from build123d import *

# Parameters (mm, degrees)
SKETCH1_W           = 164
SKETCH1_H           = 55
SKETCH1_W_2         = 15
SKETCH1_H_2         = 2.5
BOSS_EXTRUDE1_DEPTH = 3
CUT_EXTRUDE1_DEPTH  = 3
SKETCH3_R           = 1.25
CUT_EXTRUDE2_DEPTH  = 10
SKETCH4_R           = 2.5
CUT_EXTRUDE3_DEPTH  = 4
SKETCH5_R           = 1.5
CUT_EXTRUDE4_DEPTH  = 10


with BuildPart() as part:
    # Sketch1 → Boss-Extrude1 (new body)
    with BuildSketch(Plane(origin=(0, 0, 0), x_dir=(1, 0, 0), z_dir=(0, 1, 0))):
        Rectangle(SKETCH1_W, SKETCH1_H)
        with Locations((48.5, 14.5)):
            Rectangle(SKETCH1_W_2, SKETCH1_H_2, mode=Mode.SUBTRACT)
        with Locations((68.5, 14.5)):
            Rectangle(SKETCH1_W_2, SKETCH1_H_2, mode=Mode.SUBTRACT)
        with Locations((68.5, -14.5)):
            Rectangle(SKETCH1_W_2, SKETCH1_H_2, mode=Mode.SUBTRACT)
        with Locations((48.5, -14.5)):
            Rectangle(SKETCH1_W_2, SKETCH1_H_2, mode=Mode.SUBTRACT)
        with Locations((-48.5, -14.5)):
            Rectangle(SKETCH1_W_2, SKETCH1_H_2, mode=Mode.SUBTRACT)
        with Locations((-68.5, -14.5)):
            Rectangle(SKETCH1_W_2, SKETCH1_H_2, mode=Mode.SUBTRACT)
        with Locations((-68.5, 14.5)):
            Rectangle(SKETCH1_W_2, SKETCH1_H_2, mode=Mode.SUBTRACT)
        with Locations((-48.5, 14.5)):
            Rectangle(SKETCH1_W_2, SKETCH1_H_2, mode=Mode.SUBTRACT)
    extrude(amount=BOSS_EXTRUDE1_DEPTH)

    # Sketch2 → Cut-Extrude1 (cut)
    with BuildSketch(Plane(origin=(0, 3, 0), x_dir=(1, 0, 0), z_dir=(0, 1, 0))):
        with BuildLine():
            Line((-31.658505885, 2), (-8.266387648, 2))
            ThreePointArc((-8.266387648, 2), (-6.266387648, 0), (-8.266387648, -2))
            Line((-8.266387648, -2), (-31.658505885, -2))
            ThreePointArc((-31.658505885, -2), (-33.658505885, 0), (-31.658505885, 2))
        make_face()
        with BuildLine():
            Line((31.658505885, -9.856733432), (8.266387648, -9.856733432))
            ThreePointArc((8.266387648, -9.856733432), (6.266387648, -7.856733432), (8.266387648, -5.856733432))
            Line((8.266387648, -5.856733432), (31.658505885, -5.856733432))
            ThreePointArc((31.658505885, -5.856733432), (33.658505885, -7.856733432), (31.658505885, -9.856733432))
        make_face()
        with BuildLine():
            Line((-31.658505885, 9.620758334), (-8.266387648, 9.620758334))
            ThreePointArc((-8.266387648, 9.620758334), (-6.266387648, 7.620758334), (-8.266387648, 5.620758334))
            Line((-8.266387648, 5.620758334), (-31.658505885, 5.620758334))
            ThreePointArc((-31.658505885, 5.620758334), (-33.658505885, 7.620758334), (-31.658505885, 9.620758334))
        make_face()
        with BuildLine():
            Line((31.658505885, 5.620758334), (8.266387648, 5.620758334))
            ThreePointArc((8.266387648, 5.620758334), (6.266387648, 7.620758334), (8.266387648, 9.620758334))
            Line((8.266387648, 9.620758334), (31.658505885, 9.620758334))
            ThreePointArc((31.658505885, 9.620758334), (33.658505885, 7.620758334), (31.658505885, 5.620758334))
        make_face()
        with BuildLine():
            Line((-31.658505885, -5.856733432), (-8.266387648, -5.856733432))
            ThreePointArc((-8.266387648, -5.856733432), (-6.266387648, -7.856733432), (-8.266387648, -9.856733432))
            Line((-8.266387648, -9.856733432), (-31.658505885, -9.856733432))
            ThreePointArc((-31.658505885, -9.856733432), (-33.658505885, -7.856733432), (-31.658505885, -5.856733432))
        make_face()
        with BuildLine():
            Line((31.658505885, -2), (8.266387648, -2))
            ThreePointArc((8.266387648, -2), (6.266387648, 0), (8.266387648, 2))
            Line((8.266387648, 2), (31.658505885, 2))
            ThreePointArc((31.658505885, 2), (33.658505885, 0), (31.658505885, -2))
        make_face()
    extrude(amount=-CUT_EXTRUDE1_DEPTH, mode=Mode.SUBTRACT)

    # Sketch3 → Cut-Extrude2 (cut)
    with BuildSketch(Plane(origin=(0, 3, 0), x_dir=(1, 0, 0), z_dir=(0, 1, 0))):
        with Locations((18.5, -18.5)):
            Circle(SKETCH3_R)
        with Locations((-18.5, -18.5)):
            Circle(SKETCH3_R)
        with Locations((-18.5, 18.5)):
            Circle(SKETCH3_R)
        with Locations((3, 18.5)):
            Circle(SKETCH3_R)
    extrude(amount=-CUT_EXTRUDE2_DEPTH, mode=Mode.SUBTRACT)

    # Sketch4 → Cut-Extrude3 (cut, through all)
    with BuildSketch(Plane(origin=(0, 3, 0), x_dir=(1, 0, 0), z_dir=(0, 1, 0))):
        with Locations((72, -22.5)):
            Circle(SKETCH4_R)
        with Locations((62, -22.5)):
            Circle(SKETCH4_R)
        with Locations((72, 22.5)):
            Circle(SKETCH4_R)
        with Locations((62, 22.5)):
            Circle(SKETCH4_R)
        with Locations((-72, 22.5)):
            Circle(SKETCH4_R)
        with Locations((-62, 22.5)):
            Circle(SKETCH4_R)
        with Locations((-72, -22.5)):
            Circle(SKETCH4_R)
        with Locations((-62, -22.5)):
            Circle(SKETCH4_R)
    extrude(amount=-CUT_EXTRUDE3_DEPTH, mode=Mode.SUBTRACT)

    # Sketch5 → Cut-Extrude4 (cut)
    with BuildSketch(Plane.XZ):
        with Locations((52, 10)):
            Circle(SKETCH5_R)
        with Locations((62, 10)):
            Circle(SKETCH5_R)
        with Locations((62, 0)):
            Circle(SKETCH5_R)
        with Locations((52, 0)):
            Circle(SKETCH5_R)
        with Locations((52, -10)):
            Circle(SKETCH5_R)
        with Locations((62, -10)):
            Circle(SKETCH5_R)
        with Locations((-52, 10)):
            Circle(SKETCH5_R)
        with Locations((-52, 0)):
            Circle(SKETCH5_R)
        with Locations((-52, -10)):
            Circle(SKETCH5_R)
        with Locations((-62, 10)):
            Circle(SKETCH5_R)
        with Locations((-62, 0)):
            Circle(SKETCH5_R)
        with Locations((-62, -10)):
            Circle(SKETCH5_R)
    extrude(amount=-CUT_EXTRUDE4_DEPTH, mode=Mode.SUBTRACT)


solid = part.part
Could you check a few things on this model? Use its own coordinates, in mm. A direction names the side the tool comes from. Round coordinates to 2 decimals unless told otherwise and drop trailing zeros. Loops run counter-clockwise (first coordinate to the right, second up) from the corner with the lowest first, then second, coordinate; pieces in that order, holes last. Notation, with made-up numbers: (-5.75, -31.5) - (31.25, -31.5) arc R24 ccw to (31.25, -3.5) - close; hole circle Ø4 at (-30, -25.5). An arc over 180 degrees is marked (long way). Write item = value, one per line.
1) Imagine slicing it at D-D (y = 1.5). Give the number of separate pieces and of enclosed holes in the cut face, and give its area (3 significant figures).
Computed:
separate_pieces = 1
enclosed_holes = 38
area = 7,820 mm2
2) Imagine slicing it at C-C (z = 0). Please give me the cut outline in (x, y).
Computed:
outline = (-82, 0) - (-63.5, 0) - (-63.5, 3) - (-82, 3) - close; (-60.5, 0) - (-53.5, 0) - (-53.5, 3) - (-60.5, 3) - close; (-50.5, 0) - (-33.66, 0) - (-33.66, 3) - (-50.5, 3) - close; (-6.27, 0) - (6.27, 0) - (6.27, 3) - (-6.27, 3) - close; (33.66, 0) - (50.5, 0) - (50.5, 3) - (33.66, 3) - close; (53.5, 0) - (60.5, 0) - (60.5, 3) - (53.5, 3) - close; (63.5, 0) - (82, 0) - (82, 3) - (63.5, 3) - close
3) Imagine slicing it at B-B (z = 22.5). Please give me the cut outline in (x, y), and give its area (3 significant figures).
Computed:
outline = (-82, 0) - (-74.5, 0) - (-74.5, 3) - (-82, 3) - close; (-69.5, 0) - (-64.5, 0) - (-64.5, 3) - (-69.5, 3) - close; (-59.5, 0) - (59.5, 0) - (59.5, 3) - (-59.5, 3) - close; (64.5, 0) - (69.5, 0) - (69.5, 3) - (64.5, 3) - close; (74.5, 0) - (82, 0) - (82, 3) - (74.5, 3) - close
area = 432 mm2
4) Imagine slicing it at A-A (x = 42.5). Please give me the cut outline in (y, z), and give its area (3 significant figures).
Computed:
outline = (0, -27.5) - (3, -27.5) - (3, -15.75) - (0, -15.75) - close; (0, -13.25) - (3, -13.25) - (3, 13.25) - (0, 13.25) - close; (0, 15.75) - (3, 15.75) - (3, 27.5) - (0, 27.5) - close
area = 150 mm2
5) I'm going to push a flat-ended pin straight in: P1, Ø6, axis at x = 62, z = 22.5, coming from the -Y side. Where does the tip first touch, or does it pass through?
Computed:
P1 = 0
6) If we mould it in two halves opening along X, with no side actions, what happens to faces 1 (the flat face through (-82, 1, 0)), 2 (the cylindrical face through (-33.66, 1.52, -7.58)), 3 (the flat face through (-1, 3, 0))? For each: pulls with the +X half, pulls with the -X half, needs draft (parallel to the pull), parting line crosses it, or undercut.
Computed:
face_1 = pulls with the -X half
face_2 = undercut
face_3 = needs draft
7) I need wall thicknesses on line 1 along Z through (x, y) = (8, 0.9); line 2 along Z through (x, y) = (-72, 1.6); line 3 along X through (y, z) = (0.8, 18.5). Which ranges of each line are inside material? Lowest first, please. Write a range as from..to.
Computed:
line_1 = -27.5..-9.6, -5.64..-1.98, 1.98..5.87, 9.84..27.5
line_2 = -27.5..-25, -20..-15.75, -13.25..13.25, 15.75..20, 25..27.5
line_3 = -82..-19.75, -17.25..17.25, 19.75..82
8) On a 3-axis mill with a long thin cutter (end or side, diameter ignored), from which of +Z, -Z, +X, -X, +Y, -Y can I reach the whole of each face in a straight line? I mean faces 4 (the flat face through (-1, 1, -27.5)), 5 (the flat face through (-20, 2, -2)). Say none if no direction works.
Computed:
face_4 = -Z, +X, -X, +Y, -Y
face_5 = +Y, -Y
